The listing builds one solid part. Answer for the finished solid, in the listing's coordinates (mm). Face numbers are marked on the shaded views. A direction names the side the tool comes from. Give positions to 0.01 mm unless a question says otherwise; leave off trailing zeros. Write each loop counter-clockwise with the first axis right and the second up, starting at its lowest first coordinate (ties: lowest second). Pieces come first, ordered by that corner, then holes. Notation, with made-up numbers: (87, 3.5) - (105, 3.5) arc R7 ccw to (105, 12.5) - close; hole circle Ø10 at (74.5, 43.5). An arc over 180 degrees is marked (long way). Return JSON: item names as keys, results as strings.
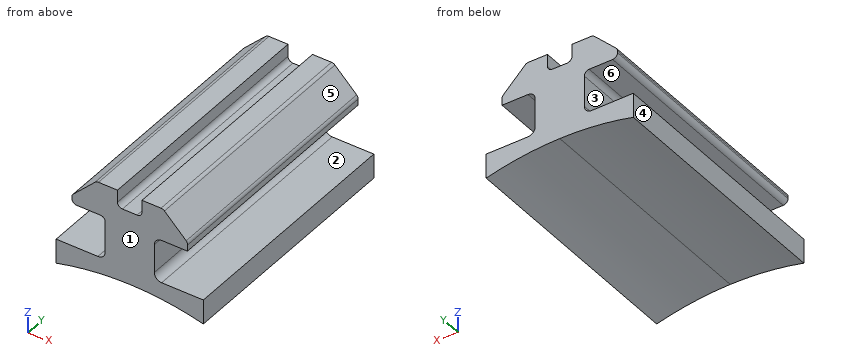
from build123d import *

# Parameters (mm, degrees)
F1_DEPTH = 10
F2_R     = 0.2
F3_R     = 0.3


# Not quite as in the source:
# - a feature names something its author has since deleted; it is built from what else it names


with BuildPart() as f1:
    # F0 (on Front) → F1 (new body)
    with BuildSketch(Plane.XZ):
        with BuildLine():
            Line((-3, 0.8663841993), (-3, -0.1336158007))
            ThreePointArc((-3, -0.1336158007), (-1.5120515098, 0.1517905158), (0, 0.2474341606))
            ThreePointArc((0, 0.2474341606), (1.5120515098, 0.1517905158), (3, -0.1336158007))
            Line((3, -0.1336158007), (3, 0.8663841993))
            Line((3, 0.8663841993), (1, 0.8663841993))
            Line((1, 0.8663841993), (1, 2.6280805469))
            Line((1, 2.6280805469), (2.3511576001, 2.6280805469))
            Line((2.3511576001, 2.6280805469), (2.363298554, 2.9764297366))
            Line((2.363298554, 2.9764297366), (1.357049332, 3.9621986704))
            Line((1.357049332, 3.9621986704), (0.5, 3.9621986704))
            Line((0.5, 3.9621986704), (0.5, 3.2621986704))
            Line((0.5, 3.2621986704), (0, 3.2621986704))
            Line((0, 3.2621986704), (-0.5, 3.2621986704))
            Line((-0.5, 3.2621986704), (-0.5, 3.9621986704))
            Line((-0.5, 3.9621986704), (-1.357049332, 3.9621986704))
            Line((-1.357049332, 3.9621986704), (-2.363298554, 2.9764297366))
            Line((-2.363298554, 2.9764297366), (-2.3511576001, 2.6280805469))
            Line((-2.3511576001, 2.6280805469), (-1, 2.6280805469))
            Line((-1, 2.6280805469), (-1, 0.8663841993))
            Line((-1, 0.8663841993), (-3, 0.8663841993))
        make_face()
    extrude(amount=F1_DEPTH)

    # F2
    f2_edges = [f1.edges().sort_by_distance(p)[0] for p in [
        (-0.5, -5, 3.262199),
        (0.5, -5, 3.262199),
        (2.363299, -5, 2.97643),
        (1.357049, -5, 3.962199),
        (-1, -5, 2.628081),
        (-2.351158, -5, 2.628081),
        (-2.363299, -5, 2.97643),
        (-1.357049, -5, 3.962199),
    ]]
    fillet(f2_edges, radius=F2_R)

    # F3
    f3_edges = [f1.edges().sort_by_distance(p)[0] for p in [
        (-1, -5, 0.866384),
        (1, -5, 0.866384),
        (1, -5, 2.628081),
    ]]
    fillet(f3_edges, radius=F3_R)


solid = f1.part
Item 1: The mould has two halves that part along Z. Classify the marked faces 4, 5 and 6: +Z half, -Z half, draft (parallel to the pull), parting line (faces both ways), or undercut.
Answer below:
{"face 4": "draft", "face 5": "+Z half", "face 6": "undercut"}
Item 2: Flat-ended cylindrical pins translate along their axes: P1, Ø0.8, axis at x = -2, y = -5.5, coming from the +Z side; P2, Ø1.4, axis at x = 2.5, y = -3.5, coming from the +Z side; P3, Ø0.5, axis at x = -1.5, y = -7, coming from the -Z side; P4, Ø1, axis at x = 2, z = 0.5, coming from the +Y side. Find the tip coordinate at first contact, or state that the pin passes through.
Answer below:
{"P1": "stops at z = 3.72", "P2": "stops at z = 3.53", "P3": "stops at z = 0.12", "P4": "stops at y = 0"}
Item 3: A cutting plane is placed at D-D on x = -0.1. Determine the outline of the cut face in (y, z).
Answer below:
{"outline": "(-10, 0.25) - (0, 0.25) - (0, 3.26) - (-10, 3.26) - close"}
Item 4: For the marked faces 1, 2 and 3, determine the directions among +Z, -Z, +X, -X, +Y, -Y from which every point of the face is accessible in a straight line to the end or side of a thin tool.
Answer below:
{"face 1": "+Z, -Z, +X, -X, -Y", "face 2": "+X, +Y, -Y", "face 3": "-X, +Y, -Y"}
Item 5: A cutting plane is placed at A-A on z = 3.7. Determine the outline of the cut face in (x, y), then the cut area to 3 significant figures.
Answer below:
{"outline": "(-1.62, -10) - (-0.5, -10) - (-0.5, 0) - (-1.62, 0) - close; (0.5, -10) - (1.62, -10) - (1.62, 0) - (0.5, 0) - close", "area": "22.5 mm²"}
Item 6: A cutting plane is placed at C-C on z = 1.75. Determine the outline of the cut face in (x, y).
Answer below:
{"outline": "(-1, -10) - (1, -10) - (1, 0) - (-1, 0) - close"}
Item 7: Consider L1, parallel to X at y = -3.75, z = 3.4; L2, parallel to X at y = -2, z = 2; L3, parallel to Z at x = -2, y = -3. Determine where each line is inside the solid, lowest interval first.
Answer below:
{"L1": "x = -1.93 to -0.49, 0.49 to 1.93", "L2": "x = -1 to 1", "L3": "z = 0.08 to 0.87, 2.63 to 3.33"}
